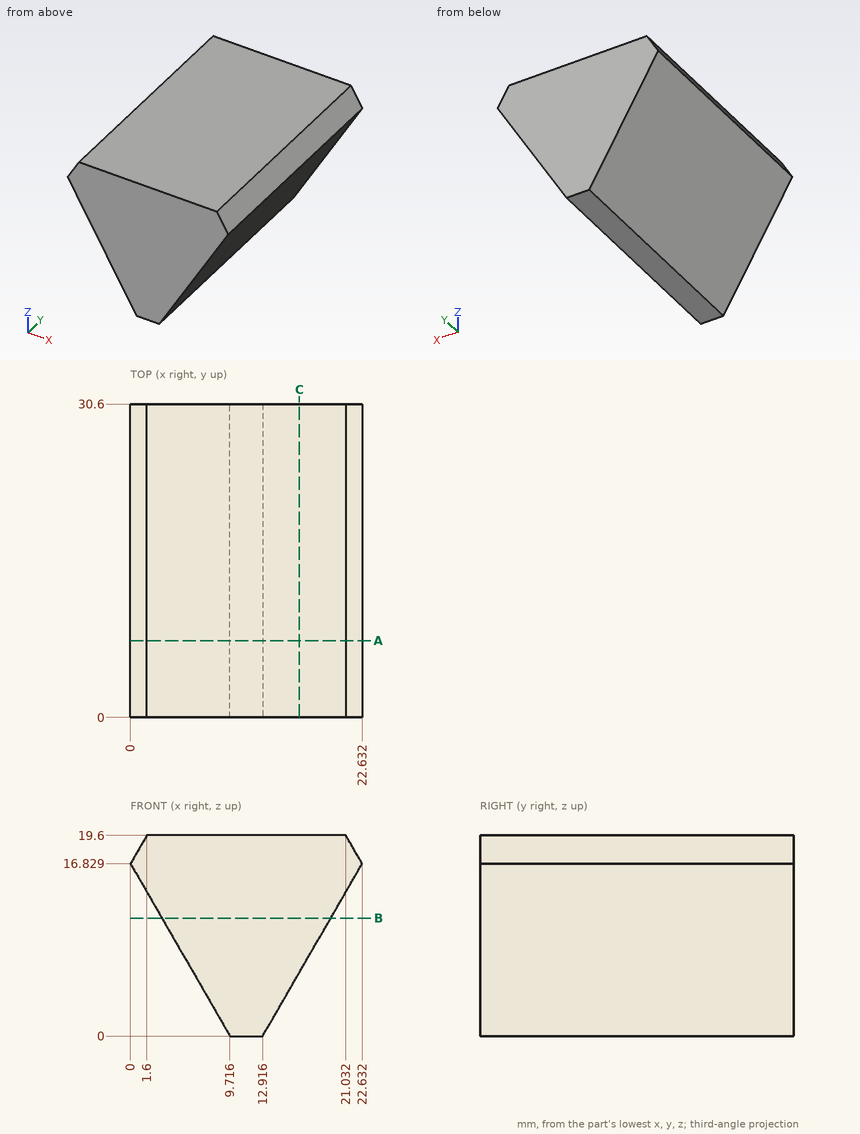
Input: dimensioned drawing with shaded views. Units: mm. Origin: part minimum x, y, z. Give positions to 0.01 mm unless a question says otherwise; leave off trailing zeros. Order: outer loops, then holes, each group sorted by start corner. A loop starts at its lowest first (then second) coordinate and runs counter-clockwise, first axis right, second up. Notation, with made-up numbers: (50.25, -38) -> (56.25, -38) arc R10 cw to (56.25, -26) -> close; hole circle Ø1 at (-6.5, -5.75). An arc over 180 degrees is marked (long way). Use a Markdown table: item, result.
1) Section query C-C, the plane x = 16.5. Return the cut outline in (y, z).
Answer list:
| item | result |
|---|---|
| outline | (0, 6.21) -> (30.6, 6.21) -> (30.6, 19.6) -> (0, 19.6) -> close |
2) Ray query, line 1 along X through (y, z) = (18.5, 11) (1 decimal); line 2 along X through (y, z) = (5.5, 9.75) (1 decimal); line 3 along Z through (x, y) = (5.75, 8.5). Return the intervals inside material, ascending. Write a range as [from, to].
Answer list:
| item | result |
|---|---|
| line 1 | [3.4, 19.3] |
| line 2 | [4.1, 18.5] |
| line 3 | [6.87, 19.6] |
3) Section query A-A, the plane y = 7.5. Return the cut outline in (x, z).
Answer list:
| item | result |
|---|---|
| outline | (0, 16.83) -> (9.72, 0) -> (12.92, 0) -> (22.63, 16.83) -> (21.03, 19.6) -> (1.6, 19.6) -> close |
4) Section query B-B, the plane z = 11.5. Return the cut outline in (x, y), then the cut area to 3 significant figures.
Answer list:
| item | result |
|---|---|
| outline | (3.08, 0) -> (19.56, 0) -> (19.56, 30.6) -> (3.08, 30.6) -> close |
| area | 504 mm² |
5) Contact query for flat-ended pins moving along their axis: P1, Ø2, axis at y = 22.5, z = 15, coming from the -X side; P2, Ø5, axis at y = 20.5, z = 6, coming from the +X side; P3, Ø6, axis at y = 26.5, z = 3.5, coming from the +X side. Output: stop coordinate, or through.
Answer list:
| item | result |
|---|---|
| P1 | x = 0.48 |
| P2 | x = 17.82 |
| P3 | x = 16.67 |
